Check sheet for the drawn part. Datum: minimum x, y, z corner. Units: mm. Coordinates: 2 decimals unless noted, no trailing zeros. Order: outer loops, then holes, each group sorted by start corner. A loop starts at its lowest first (then second) coordinate and runs counter-clockwise, first axis right, second up.
Q1. Thickness scan on line 1 (Y direction, x = 6.5, z = 2.45); line 2 (Y direction, x = 5, z = 4.7); line 3 (Y direction, x = 25.5, z = 2.7). Record the ranges inside material, lowest first.
Q2. Depth check by flat-ended pin: P1, Ø3.5, axis at x = 6.5, y = 5, coming from the +Z side (1 decimal). Enter the tip coordinate at first touch or a pass-through.
Q3. Cross-section at B-B, the plane y = 20. Record the boundary of the cut face in (x, z).
Q4. Cross-section at D-D, the plane x = 25.5. Record the boundary of the cut face in (y, z).
Q5. Draft check along X on the marked faces 1, 2, 3 and 4. Enter one of: pulls with the +X half, pulls with the -X half, needs draft (parallel to the pull), parting line crosses it, or undercut.
Q6. Cross-section at A-A, the plane x = 6.5. Record the boundary of the cut face in (y, z).
Q7. Cross-section at C-C, the plane z = 0.75. Record the boundary of the cut face in (x, y), and give its area (3 significant figures).
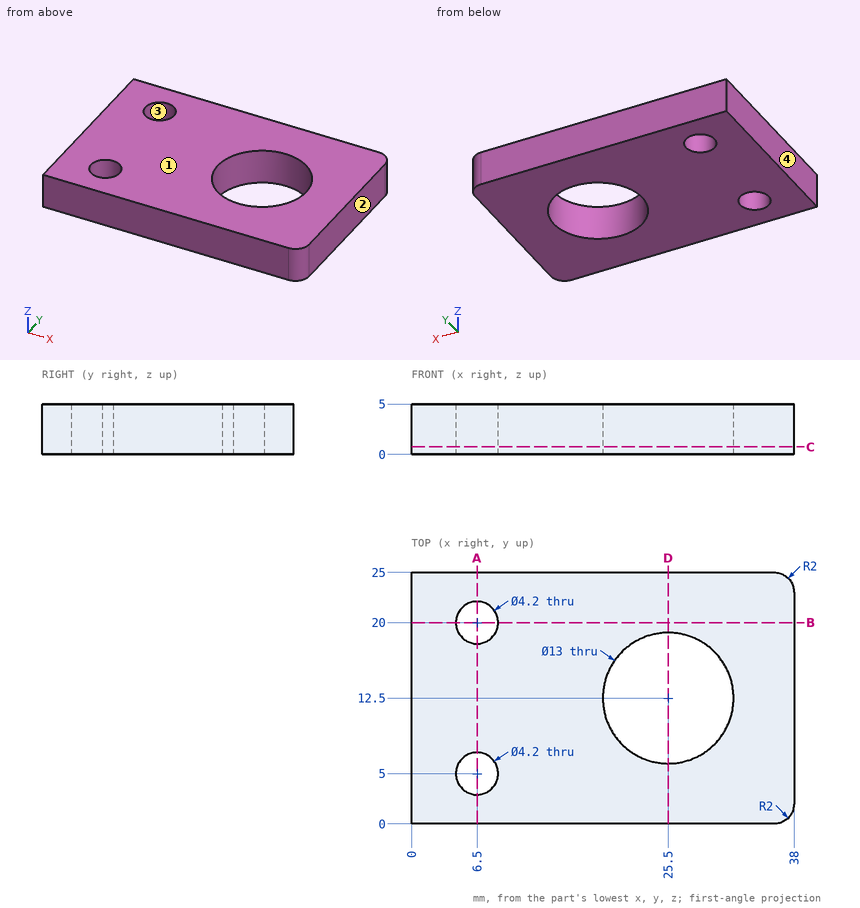
Check values:
1. line 1: y = 0 to 2.9, 7.1 to 17.9, 22.1 to 25
1. line 2: y = 0 to 3.53, 6.47 to 18.53, 21.47 to 25
1. line 3: y = 0 to 6, 19 to 25
2. P1: passes through
3. outline: (0, 0) - (4.4, 0) - (4.4, 5) - (0, 5) - close; (8.6, 0) - (38, 0) - (38, 5) - (8.6, 5) - close
4. outline: (0, 0) - (6, 0) - (6, 5) - (0, 5) - close; (19, 0) - (25, 0) - (25, 5) - (19, 5) - close
5. face 1: needs draft
5. face 2: pulls with the +X half
5. face 3: undercut
5. face 4: pulls with the -X half
6. outline: (0, 0) - (2.9, 0) - (2.9, 5) - (0, 5) - close; (7.1, 0) - (17.9, 0) - (17.9, 5) - (7.1, 5) - close; (22.1, 0) - (25, 0) - (25, 5) - (22.1, 5) - close
7. outline: (0, 0) - (36, 0) arc R2 ccw to (38, 2) - (38, 23) arc R2 ccw to (36, 25) - (0, 25) - close; hole circle Ø4.2 at (6.5, 5); hole circle Ø4.2 at (6.5, 20); hole circle Ø13 at (25.5, 12.5)
7. area: 788 mm2
